The model under review builds one solid part; all positions refer to its coordinate system, in mm. A direction names the side the tool comes from. Round coordinates to 2 decimals unless told otherwise and drop trailing zeros. Write each loop counter-clockwise with the first axis right and the second up, starting at its lowest first coordinate (ties: lowest second). Pieces come first, ordered by that corner, then holes. Notation, with made-up numbers: M 66.5,-34 L 75.5,-34 A33 cw 75.5,2 Z; hole C 78.5,12 d3. An arc over 180 degrees is marked long. One line per item, written item: value. Start each with the question number.
1) For P1, Ø15.5, axis at x = 0, z = 13, coming from the +Y side, flat-tipped, find the tip position at first contact; note if it passes through.
2) Wall thickness on probe 1 along Z at (x, y) = (7.5, -20.5); probe 2 along Y at (x, z) = (6.5, 25): over which ranges is each line inside the solid? List them lowest first.
3) Take a section at B-B, the plane x = -6. Write out the cut boundary in (y, z), and give its area (3 significant figures).
4) Take a section at A-A, the plane y = 37. Write out the cut boundary in (x, z), and give its area (3 significant figures).
5) Mouldability with a two-part tool opening along X and no side actions: class faces 1 (the face through (-1, 1, 0)), 2 (the face through (40.598, 1, 32)), 3 (the face through (43.138, -1, 17)) as +X half, -X half, draft (parallel to the pull), parting line (faces both ways), or undercut.
6) Tool access review of faces 4 (the face through (-1, 1, 34.798)), 5 (the face through (-1, 2, 31.496)), 6 (the face through (-1, 67.768, 16)): name each direction out of +Z, -Z, +X, -X, +Y, -Y from which nothing blocks a thin tool from reaching the whole face with its end or side.
from build123d import *

# Parameters (mm, degrees)
F0_W     = 86.276724
F0_H     = 136.701972
F1_DEPTH = 34.798
F2_T     = -2.54
F3_W     = 84.527872
F3_H     = 135.53606
F4_DEPTH = 31.496


with BuildPart() as f1:
    # F0 (on Top) → F1 (new body)
    with BuildSketch(Plane.XY):
        Rectangle(F0_W, F0_H)
    extrude(amount=F1_DEPTH)

    # F2
    f2_openings = [f1.faces().sort_by_distance(p)[0] for p in [
        (0, 0, 0),
        (0, 68.350986, 17.399),
    ]]
    offset(amount=F2_T, openings=f2_openings)

    # F3 (on Top) → F4 (join)
    with BuildSketch(Plane.XY):
        Rectangle(F3_W, F3_H)
    extrude(amount=F4_DEPTH)


solid = f1.part
Checked values:
1. P1: stops at y = 67.77
2. probe 1: z = 0 to 31.5, 32.26 to 34.8
2. probe 2: y = -68.35 to 67.77
3. outline: M -68.35,0 L 67.77,0 L 67.77,31.5 L -65.81,31.5 L -65.81,32.26 L 68.35,32.26 L 68.35,34.8 L -68.35,34.8 Z
3. area: 4,640 mm2
4. outline: M -43.14,0 L 43.14,0 L 43.14,34.8 L -43.14,34.8 Z; hole M -40.6,31.5 L 40.6,31.5 L 40.6,32.26 L -40.6,32.26 Z
4. area: 2,940 mm2
5. face 1: draft
5. face 2: undercut
5. face 3: +X half
6. face 4: +Z, +X, -X, +Y, -Y
6. face 5: +Y
6. face 6: -Z, +Y
